For this review, take the finished solid that the model builds, in its own axes (mm). A direction names the side the tool comes from. Coordinates: 2 decimals unless noted, no trailing zeros. Loops run counter-clockwise (first coordinate to the right, second up) from the corner with the lowest first, then second, coordinate; pieces in that order, holes last. Notation, with made-up numbers: (-40, 1.25) - (8, 1.25) arc R18 cw to (8, 16.25) - close; hole circle Ø5 at (7.5, 61). An arc over 180 degrees is marked (long way). Use one line per item in the form item = value. Start each with the question number.
1. Add section D-D on y = 3. Give the boundary of the cut face in (x, z), and give its area (3 significant figures).
2. Add section A-A on z = 0. Give the boundary of the cut face in (x, y), and give its area (3 significant figures).
3. Add section B-B on x = -8. Give the boundary of the cut face in (y, z).
4. Add section C-C on z = -8. Give the boundary of the cut face in (x, y).
5. Machinability: for faces 1 (the face through (-10.74, 0.99, -2.38)), 2 (the face through (-5, 2, 2)), which of the approach directions +Z, -Z, +X, -X, +Y, -Y give a long, thin tool a straight path to every point of the face, cutting with its end or side? Answer none if there is none.
6. Draft analysis for pull direction X (two halves, no side actions). For faces 3 (the face through (1.5, 6.93, 4.77)), 4 (the face through (-3.3, 12, -0.1)), 5 (the face through (0.07, 1.01, -9.5)), state which applies: +X half, -X half, draft (parallel to the pull), parting line (faces both ways), or undercut.
7. For pin 1 Ø1.5 at (y, z) = (5.5, 2.5) entering from -X; pin 2 Ø2 at (y, z) = (9.5, 7.5) entering from -X; pin 3 Ø4 at (y, z) = (8, 0) entering from +X; pin 4 Ø3 at (y, z) = (8, 0) entering from -X, all flat-tipped, find the tip position at first contact; note any pin that passes through.
8. To check wall thickness, follow probe 1 along X at (y, z) = (6, 0); probe 2 along X at (y, z) = (1.3, 8); probe 3 along Y at (x, z) = (-4.4, 0). State the ranges of each line that lie inside material, in increasing order.
```python
from build123d import *

# Parameters (mm, degrees)
SKETCH_1_R               = 11
EXTRUDE_1_DEPTH          = 2
SKETCH_2_R               = 5
EXTRUDE_2_DEPTH          = 10
SKETCH_3_R               = 3
CUT_EXTRUDE_1_DEPTH      = 20.646882704
SKETCH_4_R               = 1.5
CUT_EXTRUDE_2_DEPTH      = 10
CUT_EXTRUDE_3_DEPTH      = 20.646882704
CUT_EXTRUDE_3_DEPTH_BACK = 20.646882704
SKETCH_5_R               = 1.2


with BuildPart() as part:
    # 草图1 → 凸台-拉伸1 (new body)
    with BuildSketch(Plane(origin=(0, 0, 0), x_dir=(1, 0, 0), z_dir=(0, 1, 0))):
        with Locations(Location((0, 0, 0), (0, 0, 270))):
            Circle(SKETCH_1_R)
    extrude(amount=EXTRUDE_1_DEPTH)

    # 草图2 → 凸台-拉伸2 (add)
    with BuildSketch(Plane(origin=(0, 2, 0), x_dir=(1, 0, 0), z_dir=(0, 1, 0))):
        with Locations(Location((0, 0, 0), (0, 0, 270))):
            Circle(SKETCH_2_R)
    extrude(amount=EXTRUDE_2_DEPTH)

    # 草图3 → 切除-拉伸1 (cut, through all)
    with BuildSketch(Plane(origin=(0, 12, 0), x_dir=(1, 0, 0), z_dir=(0, 1, 0))):
        with Locations(Location((0, 0, 0), (0, 0, 270))):
            Circle(SKETCH_3_R)
    extrude(amount=-CUT_EXTRUDE_1_DEPTH, mode=Mode.SUBTRACT)

    # 草图4 → 切除-拉伸2 (cut)
    with BuildSketch(Plane(origin=(0, 2, 0), x_dir=(1, 0, 0), z_dir=(0, 1, 0))):
        with Locations(Location((0, 8, 0), (0, 0, 270))):
            Circle(SKETCH_4_R)
        with Locations(Location((8, 0, 0), (0, 0, 270))):
            Circle(SKETCH_4_R)
        with Locations(Location((0, -8, 0), (0, 0, 270))):
            Circle(SKETCH_4_R)
        with Locations(Location((-8, 0, 0), (0, 0, 270))):
            Circle(SKETCH_4_R)
    extrude(amount=-CUT_EXTRUDE_2_DEPTH, mode=Mode.SUBTRACT)

    # 草图5 → 切除-拉伸3 (cut, two sides: drawn at the far end of the back side and taken through both)
    with BuildSketch(Plane(origin=(0, 0, 0), x_dir=(0, 0, -1), z_dir=(1, 0, 0)).offset(-CUT_EXTRUDE_3_DEPTH_BACK)):
        with Locations((0, 8)):
            Circle(SKETCH_5_R)
    extrude(amount=CUT_EXTRUDE_3_DEPTH + CUT_EXTRUDE_3_DEPTH_BACK, mode=Mode.SUBTRACT)


solid = part.part
```
Conclusion:
q1.outline = circle Ø10 at (0, 0); hole circle Ø6 at (0, 0)
q1.area = 50.3 mm^2
q2.outline = (-11, 0) - (-9.5, 0) - (-9.5, 2) - (-11, 2) - close; (-6.5, 0) - (-3, 0) - (-3, 6.8) - (-5, 6.8) - (-5, 2) - (-6.5, 2) - close; (-5, 9.2) - (-3, 9.2) - (-3, 12) - (-5, 12) - close; (3, 0) - (6.5, 0) - (6.5, 2) - (5, 2) - (5, 6.8) - (3, 6.8) - close; (3, 9.2) - (5, 9.2) - (5, 12) - (3, 12) - close; (9.5, 0) - (11, 0) - (11, 2) - (9.5, 2) - close
q2.area = 50.4 mm^2
q3.outline = (0, -7.55) - (2, -7.55) - (2, -1.5) - (0, -1.5) - close; (0, 1.5) - (2, 1.5) - (2, 7.55) - (0, 7.55) - close
q4.outline = (-7.55, 0) - (-1.5, 0) - (-1.5, 2) - (-7.55, 2) - close; (1.5, 0) - (7.55, 0) - (7.55, 2) - (1.5, 2) - close
q5.face_1 = +Y, -Y
q5.face_2 = +Y
q6.face_3 = parting line
q6.face_4 = draft
q6.face_5 = undercut
q7.pin_1 = -4.68
q7.pin_2 = through
q7.pin_3 = 5
q7.pin_4 = -5
q8.probe_1 = -5 to -3, 3 to 5
q8.probe_2 = -7.55 to -1.5, 1.5 to 7.55
q8.probe_3 = 0 to 6.8, 9.2 to 12
